Geometry: final body of the model. Coordinates: model frame, mm. Give positions to 0.01 mm unless a question says otherwise; leave off trailing zeros. Loops run counter-clockwise (first coordinate to the right, second up) from the corner with the lowest first, then second, coordinate; pieces in that order, holes last. Notation, with made-up numbers: (62, 33) - (88, 33) arc R32 ccw to (88, 65) - close; hole circle Ø5 at (-8.75, 2). An arc over 180 degrees is marked (long way). Use one line per item in the form item = value.
```python
from build123d import *

# Parameters (mm, degrees)
SKETCH_1_W                  = 5
SKETCH_1_H                  = 46.025
CUT_EXTRUDE_1_DEPTH         = 6
CUT_EXTRUDE_2_DEPTH         = 6
CUT_EXTRUDE_3_DEPTH         = 6
CUT_EXTRUDE_4_DEPTH         = 6
CUT_EXTRUDE_5_DEPTH         = 6
CUT_EXTRUDE_6_DEPTH         = 6
CUT_EXTRUDE_7_DEPTH         = 6
CUT_EXTRUDE_8_DEPTH         = 6
CUT_EXTRUDE_9_DEPTH         = 6
CUT_EXTRUDE_10_DEPTH        = 6
CUT_EXTRUDE_11_DEPTH        = 6
CUT_EXTRUDE_12_DEPTH        = 6
HOLE_WIZARD_17_0_17_1_D     = 17
HOLE_WIZARD_17_0_17_1_DEPTH = 5
HOLE_WIZARD_3_0_3_1_D       = 3.1
HOLE_WIZARD_3_0_3_1_DEPTH   = 5
CHAMFER_1_SIZE              = 1.5


with BuildPart() as part:
    # 草图1 → 旋转1 (revolve)
    with BuildSketch(Plane.XY):
        with Locations((0, 23.0125)):
            Rectangle(SKETCH_1_W, SKETCH_1_H)
    revolve(axis=Axis((-2.5, 0, 0), (1, 0, 0)))

    # 草图2 → 切除-拉伸1 (cut, through all)
    with BuildSketch(Plane(origin=(2.5, 0, 0), x_dir=(0, 0, -1), z_dir=(1, 0, 0))):
        with BuildLine():
            ThreePointArc((20.169819251, -5.846228817), (18.186533479, -10.5), (15.147892297, -14.544461453))
            ThreePointArc((15.147892297, -14.544461453), (15.277198907, -20.907108685), (21.639846139, -20.777802075))
            ThreePointArc((21.639846139, -20.777802075), (25.980762114, -15), (28.814027502, -8.351755453))
            ThreePointArc((28.814027502, -8.351755453), (25.744686694, -2.776888009), (20.169819251, -5.846228817))
        make_face()
    extrude(amount=-CUT_EXTRUDE_1_DEPTH, mode=Mode.SUBTRACT)

    # 草图3 → 切除-拉伸2 (cut, through all)
    with BuildSketch(Plane(origin=(2.5, 0, 0), x_dir=(0, 0, -1), z_dir=(1, 0, 0))):
        with BuildLine():
            ThreePointArc((5.021926954, -20.39069027), (0, -21), (-5.021926954, -20.39069027))
            ThreePointArc((-5.021926954, -20.39069027), (-10.467487787, -23.683996694), (-7.174181363, -29.129557528))
            ThreePointArc((-7.174181363, -29.129557528), (0, -30), (7.174181363, -29.129557528))
            ThreePointArc((7.174181363, -29.129557528), (10.467487787, -23.683996694), (5.021926954, -20.39069027))
        make_face()
    extrude(amount=-CUT_EXTRUDE_2_DEPTH, mode=Mode.SUBTRACT)

    # 草图4 → 切除-拉伸3 (cut, through all)
    with BuildSketch(Plane(origin=(2.5, 0, 0), x_dir=(0, 0, -1), z_dir=(1, 0, 0))):
        with BuildLine():
            ThreePointArc((-15.147892297, -14.544461453), (-18.186533479, -10.5), (-20.169819251, -5.846228817))
            ThreePointArc((-20.169819251, -5.846228817), (-25.744686694, -2.776888009), (-28.814027502, -8.351755453))
            ThreePointArc((-28.814027502, -8.351755453), (-25.980762114, -15), (-21.639846139, -20.777802075))
            ThreePointArc((-21.639846139, -20.777802075), (-15.277198907, -20.907108685), (-15.147892297, -14.544461453))
        make_face()
    extrude(amount=-CUT_EXTRUDE_3_DEPTH, mode=Mode.SUBTRACT)

    # 草图5 → 切除-拉伸4 (cut, through all)
    with BuildSketch(Plane(origin=(2.5, 0, 0), x_dir=(0, 0, -1), z_dir=(1, 0, 0))):
        with BuildLine():
            ThreePointArc((15.147892297, 14.544461453), (18.186533479, 10.5), (20.169819251, 5.846228817))
            ThreePointArc((20.169819251, 5.846228817), (25.744686694, 2.776888009), (28.814027502, 8.351755453))
            ThreePointArc((28.814027502, 8.351755453), (25.980762114, 15), (21.639846139, 20.777802075))
            ThreePointArc((21.639846139, 20.777802075), (15.277198907, 20.907108685), (15.147892297, 14.544461453))
        make_face()
    extrude(amount=-CUT_EXTRUDE_4_DEPTH, mode=Mode.SUBTRACT)

    # 草图6 → 切除-拉伸5 (cut, through all)
    with BuildSketch(Plane(origin=(2.5, 0, 0), x_dir=(0, 0, -1), z_dir=(1, 0, 0))):
        with BuildLine():
            ThreePointArc((-20.169819251, 5.846228817), (-18.186533479, 10.5), (-15.147892297, 14.544461453))
            ThreePointArc((-15.147892297, 14.544461453), (-15.277198907, 20.907108685), (-21.639846139, 20.777802075))
            ThreePointArc((-21.639846139, 20.777802075), (-25.980762114, 15), (-28.814027502, 8.351755453))
            ThreePointArc((-28.814027502, 8.351755453), (-25.744686694, 2.776888009), (-20.169819251, 5.846228817))
        make_face()
    extrude(amount=-CUT_EXTRUDE_5_DEPTH, mode=Mode.SUBTRACT)

    # 草图7 → 切除-拉伸6 (cut, through all)
    with BuildSketch(Plane(origin=(2.5, 0, 0), x_dir=(0, 0, -1), z_dir=(1, 0, 0))):
        with BuildLine():
            ThreePointArc((5.021926954, 20.39069027), (10.467487787, 23.683996694), (7.174181363, 29.129557528))
            ThreePointArc((7.174181363, 29.129557528), (0, 30), (-7.174181363, 29.129557528))
            ThreePointArc((-7.174181363, 29.129557528), (-10.467487787, 23.683996694), (-5.021926954, 20.39069027))
            ThreePointArc((-5.021926954, 20.39069027), (0, 21), (5.021926954, 20.39069027))
        make_face()
    extrude(amount=-CUT_EXTRUDE_6_DEPTH, mode=Mode.SUBTRACT)

    # 草图8 → 切除-拉伸7 (cut, through all)
    with BuildSketch(Plane(origin=(2.5, 0, 0), x_dir=(0, 0, -1), z_dir=(1, 0, 0))):
        with BuildLine():
            ThreePointArc((-22.897786978, 29.063574308), (-22.647822626, 31.170115981), (-24.7543643, 31.420080332))
            ThreePointArc((-24.7543643, 31.420080332), (-34.641016151, 20), (-39.587769907, 5.727868172))
            ThreePointArc((-39.587769907, 5.727868172), (-38.318023592, 4.028531744), (-36.618687164, 5.298278059))
            ThreePointArc((-36.618687164, 5.298278059), (-32.04293994, 18.5), (-22.897786978, 29.063574308))
        make_face()
    extrude(amount=-CUT_EXTRUDE_7_DEPTH, mode=Mode.SUBTRACT)

    # 草图9 → 切除-拉伸8 (cut, through all)
    with BuildSketch(Plane(origin=(2.5, 0, 0), x_dir=(0, 0, -1), z_dir=(1, 0, 0))):
        with BuildLine():
            ThreePointArc((-36.618687164, -5.298278059), (-38.318023592, -4.028531744), (-39.587769907, -5.727868172))
            ThreePointArc((-39.587769907, -5.727868172), (-34.641016151, -20), (-24.7543643, -31.420080332))
            ThreePointArc((-24.7543643, -31.420080332), (-22.647822626, -31.170115981), (-22.897786978, -29.063574308))
            ThreePointArc((-22.897786978, -29.063574308), (-32.04293994, -18.5), (-36.618687164, -5.298278059))
        make_face()
    extrude(amount=-CUT_EXTRUDE_8_DEPTH, mode=Mode.SUBTRACT)

    # 草图10 → 切除-拉伸9 (cut, through all)
    with BuildSketch(Plane(origin=(2.5, 0, 0), x_dir=(0, 0, -1), z_dir=(1, 0, 0))):
        with BuildLine():
            ThreePointArc((-13.720900186, -34.361852367), (-15.670200965, -35.198647725), (-14.833405607, -37.147948505))
            ThreePointArc((-14.833405607, -37.147948505), (0, -40), (14.833405607, -37.147948505))
            ThreePointArc((14.833405607, -37.147948505), (15.670200965, -35.198647725), (13.720900186, -34.361852367))
            ThreePointArc((13.720900186, -34.361852367), (0, -37), (-13.720900186, -34.361852367))
        make_face()
    extrude(amount=-CUT_EXTRUDE_9_DEPTH, mode=Mode.SUBTRACT)

    # 草图11 → 切除-拉伸10 (cut, through all)
    with BuildSketch(Plane(origin=(2.5, 0, 0), x_dir=(0, 0, -1), z_dir=(1, 0, 0))):
        with BuildLine():
            ThreePointArc((13.720900186, 34.361852367), (15.670200965, 35.198647725), (14.833405607, 37.147948505))
            ThreePointArc((14.833405607, 37.147948505), (0, 40), (-14.833405607, 37.147948505))
            ThreePointArc((-14.833405607, 37.147948505), (-15.670200965, 35.198647725), (-13.720900186, 34.361852367))
            ThreePointArc((-13.720900186, 34.361852367), (0, 37), (13.720900186, 34.361852367))
        make_face()
    extrude(amount=-CUT_EXTRUDE_10_DEPTH, mode=Mode.SUBTRACT)

    # 草图12 → 切除-拉伸11 (cut, through all)
    with BuildSketch(Plane(origin=(2.5, 0, 0), x_dir=(0, 0, -1), z_dir=(1, 0, 0))):
        with BuildLine():
            ThreePointArc((22.897786978, -29.063574308), (22.647822626, -31.170115981), (24.7543643, -31.420080332))
            ThreePointArc((24.7543643, -31.420080332), (34.641016151, -20), (39.587769907, -5.727868172))
            ThreePointArc((39.587769907, -5.727868172), (38.318023592, -4.028531744), (36.618687164, -5.298278059))
            ThreePointArc((36.618687164, -5.298278059), (32.04293994, -18.5), (22.897786978, -29.063574308))
        make_face()
    extrude(amount=-CUT_EXTRUDE_11_DEPTH, mode=Mode.SUBTRACT)

    # 草图13 → 切除-拉伸12 (cut, through all)
    with BuildSketch(Plane.ZY.offset(2.5)):
        with BuildLine():
            ThreePointArc((-39.587769907, 5.727868172), (-38.318023592, 4.028531744), (-36.618687164, 5.298278059))
            ThreePointArc((-36.618687164, 5.298278059), (-32.04293994, 18.5), (-22.897786978, 29.063574308))
            ThreePointArc((-22.897786978, 29.063574308), (-22.647822626, 31.170115981), (-24.7543643, 31.420080332))
            ThreePointArc((-24.7543643, 31.420080332), (-34.641016151, 20), (-39.587769907, 5.727868172))
        make_face()
    extrude(amount=-CUT_EXTRUDE_12_DEPTH, mode=Mode.SUBTRACT)

    # Ø17.0 (17) 直径孔1
    with Locations(Plane(origin=(2.5, 0, 0), x_dir=(0, 0, -1), z_dir=(1, 0, 0))):
        with Locations((0, 0)):
            Hole(HOLE_WIZARD_17_0_17_1_D / 2, depth=HOLE_WIZARD_17_0_17_1_DEPTH)

    # Ø3.0 (3) 直径孔1
    with Locations(Plane(origin=(2.5, 0, 0), x_dir=(0, 0, -1), z_dir=(1, 0, 0))):
        with Locations((-14, 0), (-7, 12.124355653), (7, 12.124355653), (14, 0), (7, -12.124355653), (-7, -12.124355653), (19.25, -33.341978046), (19.25, 33.341978046), (-38.5, 0), (38.5, 0), (-19.25, -33.341978046), (-19.25, 33.341978046)):
            Hole(HOLE_WIZARD_3_0_3_1_D / 2, depth=HOLE_WIZARD_3_0_3_1_DEPTH)

    # 倒角1
    chamfer_1_edges = [part.edges().sort_by_distance(p)[0] for p in [
        (2.5, -12.124355653, 5.45),
        (2.5, -12.124355653, -8.55),
        (2.5, 0, -15.55),
        (2.5, 12.124355653, -8.55),
        (2.5, 12.124355653, 5.45),
        (2.5, 0, 12.45),
    ]]
    chamfer(chamfer_1_edges, length=CHAMFER_1_SIZE)


solid = part.part
```
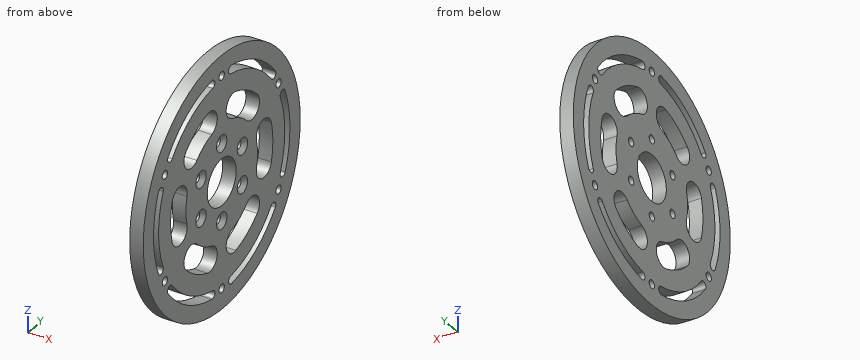
(1) Material intervals for L1, parallel to Z at x = 1.95, y = 9; L2, parallel to Z at x = 0.7, y = 7.5; L3, parallel to Z at x = -0.6, y = -32, sorted ascending. Write a range as from..to.
Solution:
L1 = -45.14..-38.97, -35.89..-28.62, -18.97..18.97, 28.62..35.89, 38.97..45.14
L2 = -45.41..-39.29, -36.23..-28.97, -19.62..-4, 4..19.62, 28.97..36.23, 39.29..45.41
L3 = -33.08..-20.03, -18.47..18.47, 20.03..33.08
(2) Cut plane C-C (z = 34). Return the cut outline in (x, y), plus the area to 3 significant figures.
Solution:
outline = (-2.5, -31.02) - (2.5, -31.02) - (2.5, -21.07) - (-2.5, -21.07) - close; (-2.5, -14.59) - (2.5, -14.59) - (2.5, 14.59) - (-2.5, 14.59) - close; (-2.5, 21.07) - (2.5, 21.07) - (2.5, 31.02) - (-2.5, 31.02) - close
area = 245 mm2
(3) Cut plane A-A (z = 0). Return the cut outline in (x, y) (3 decimals), plus the area to 3 significant figures.
Solution:
outline = (-2.5, -46.025) - (2.5, -46.025) - (2.5, -40) - (-2.5, -40) - close; (-2.5, -37) - (2.5, -37) - (2.5, -30) - (-2.5, -30) - close; (-2.5, -21) - (2.5, -21) - (2.5, -8.5) - (-2.5, -8.5) - close; (-2.5, 8.5) - (2.5, 8.5) - (2.5, 21) - (-2.5, 21) - close; (-2.5, 30) - (2.5, 30) - (2.5, 37) - (-2.5, 37) - close; (-2.5, 40) - (2.5, 40) - (2.5, 46.025) - (-2.5, 46.025) - close
area = 255 mm2
(4) Cut plane B-B (y = 23.5). Return the cut outline in (x, z).
Solution:
outline = (-2.5, -39.57) - (2.5, -39.57) - (2.5, -32.37) - (-2.5, -32.37) - close; (-2.5, -28.58) - (2.5, -28.58) - (2.5, -10.42) - (-2.5, -10.42) - close; (-2.5, 10.42) - (2.5, 10.42) - (2.5, 28.58) - (-2.5, 28.58) - close; (-2.5, 32.37) - (2.5, 32.37) - (2.5, 39.57) - (-2.5, 39.57) - close
(5) Cut plane D-D (y = -25). Return the cut outline in (x, z), plus the area to 3 significant figures.
Solution:
outline = (-2.5, -38.64) - (2.5, -38.64) - (2.5, -31.22) - (-2.5, -31.22) - close; (-2.5, -27.28) - (2.5, -27.28) - (2.5, -10.59) - (-2.5, -10.59) - close; (-2.5, 10.59) - (2.5, 10.59) - (2.5, 27.28) - (-2.5, 27.28) - close; (-2.5, 31.22) - (2.5, 31.22) - (2.5, 38.64) - (-2.5, 38.64) - close
area = 241 mm2
(6) Pin query (flat end, axial travel): P1, Ø2, axis at x = -1.5, z = -24, coming from the -Y side; P2, Ø3.5, axis at y = 0, z = -14, coming from the +X side; P3, Ø3, axis at y = -12.12, z = 7, coming from the +X side. Return the tip coordinate at first contact, or that it passes through.
Solution:
P1 = -39.87
P2 = 1.2
P3 = through
